Autodesk Inventor part; units mm, degrees
ref_plane "YZ Plane" through (0, 0, 0) normal (1, 0, 0) x (0, 1, 0)
ref_plane "XZ Plane" through (0, 0, 0) normal (0, 1, 0) x (-1, 0, 0)
ref_plane "XY Plane" through (0, 0, 0) normal (0, 0, 1) x (1, 0, 0)
sketch "Sketch1" plane through (0, 0, 0) normal (0, 0, 1) x (1, 0, 0)
  line L0 (0, 0) -> (3.175, 0)
  line L1 (3.175, 0) -> (3.175, 10)
  line L2 (3.175, 10) -> (0, 10)
  line L3 (0, 10) -> (0, 0)
  dimension "d0" = 3.175
  dimension "d1" = 10
revolve "Revolution1" add sketch "Sketch1" angle 360 about axis through (0, 10, 0) along (0, -1, 0)
shell "Shell1" thickness 0.5 removed faces 1 at (0.8826, 10, -0.0433)
thread "Thread1"
sketch "Sketch2" plane through (0, 0, 0) normal (0, -1, 0) x (1, 0, 0)
  line L0 (0, 4.6188) -> (4, 2.3094)
  line L1 (4, 2.3094) -> (4, -2.3094)
  line L2 (4, -2.3094) -> (0, -4.6188)
  line L3 (0, -4.6188) -> (-4, -2.3094)
  line L4 (-4, -2.3094) -> (-4, 2.3094)
  line L5 (-4, 2.3094) -> (0, 4.6188)
  point P0 (0, 0)
  point P1 (0, 0)
  dimension "d6" = 8
extrude "Extrusion1" add sketch "Sketch2" along normal blind 3.4
properties part number "W9011M COAXIAL CONNECTOR"
Check sheet for the modelled part. Datum: model origin and axes. Units: mm. A direction names the side the tool comes from. Round coordinates to 2 decimals unless told otherwise and drop trailing zeros. Write each loop counter-clockwise with the first axis right and the second up, starting at its lowest first coordinate (ties: lowest second). Pieces come first, ordered by that corner, then holes. Notation, with made-up numbers: M 76.5,19.25 L 103.5,19.25 A19 cw 103.5,44.25 Z; hole C 32.25,-40 d4. An arc over 180 degrees is marked long. Write item = value, one per line. Start each with the question number.
1. Section check C-C, the plane y = 6.5. Record the cut outline in (x, z) (3 decimals), then the cut area to 3 significant figures.
2. Tool access check on faces 4 (the flat face through (-4, -2, 0)), 5 (the cylindrical face through (-0.69, 5.07, 3.1)). Record the directions out of +Z, -Z, +X, -X, +Y, -Y that give a thin tool (end or side, any length) a straight path to the whole face; none if there is none.
3. Section check B-B, the plane x = 1.5. Record the cut outline in (y, z), then the cut area to 3 significant figures.
4. Gauge pin test, flat ends, axial feed: pin 1 (3 mm diameter, centred on y = 8, z = 0, fed in from +X) (3 decimals); pin 2 (1.6 mm diameter, centred on x = 1.5, z = -1, fed in from +Y); pin 3 (1 mm diameter, centred on x = 2.5, y = 5.5, fed in from -Z). Record the tip position at first contact, or that the pin passes through.
5. Section check A-A, the plane z = 0. Record the cut outline in (x, y) (3 decimals), then the cut area to 3 significant figures.
6. Release check for a two-part mould opening along X. For faces 1 (the flat face through (2.028, -1.676, -3.448)), 2 (the flat face through (-2.028, -1.676, 3.448)), 3 (the flat face through (0, 0.5, 0)) record: pulls with the +X half, pulls with the -X half, needs draft (parallel to the pull), parting line crosses it, or undercut.
7. Section check D-D, the plane x = 3. Record the cut outline in (y, z).
8. Scan lines: line 1 (Z direction, x = 0, y = 2.75) (3 decimals); line 2 (Z direction, x = -2.25, y = 3); line 3 (Y direction, x = 0.5, z = 1.5). Record each from-to range of solid material in increasing order. Write a range as [from, to].
Results found:
q1.outline = C 0,0 d6.35; hole C 0,0 d5.35
q1.area = 9.19 mm^2
q2.face_4 = +Z, -Z, -X, +Y, -Y
q2.face_5 = +Y
q3.outline = M -3.4,-3.75 L 0,-3.75 L 0,-2.8 L 10,-2.8 L 10,-2.21 L 0.5,-2.21 L 0.5,2.21 L 10,2.21 L 10,2.8 L 0,2.8 L 0,3.75 L -3.4,3.75 Z
q3.area = 39.4 mm^2
q4.pin_1 = 3.175
q4.pin_2 = 0.5
q4.pin_3 = -2.47
q5.outline = M -4,-3.4 L 4,-3.4 L 4,0 L 3.175,0 L 3.175,10 L 2.675,10 L 2.675,0.5 L -2.675,0.5 L -2.675,10 L -3.175,10 L -3.175,0 L -4,0 Z
q5.area = 39.9 mm^2
q6.face_1 = pulls with the +X half
q6.face_2 = pulls with the -X half
q6.face_3 = undercut
q7.outline = M -3.4,-2.89 L 0,-2.89 L 0,-1.04 L 10,-1.04 L 10,1.04 L 0,1.04 L 0,2.89 L -3.4,2.89 Z
q8.line_1 = [-3.175, -2.675], [2.675, 3.175]
q8.line_2 = [-2.24, -1.45], [1.45, 2.24]
q8.line_3 = [-3.4, 0.5]
